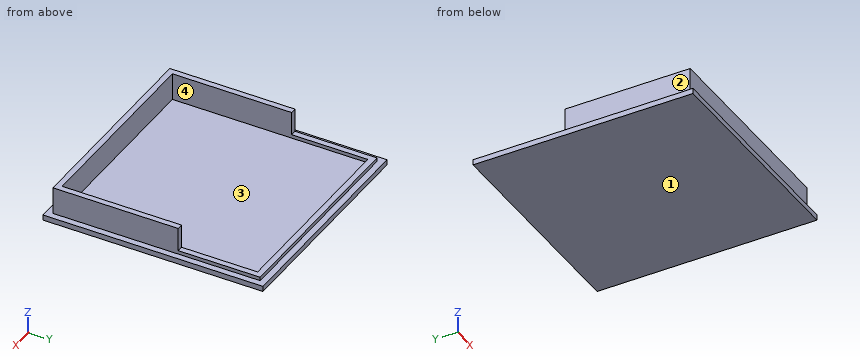
```python
from build123d import *

# Parameters (mm, degrees)
F0_W     = 48.4
F0_H     = 48.4
F3_DEPTH = 1.2
F4_DEPTH = 7.2
F5_DEPTH = 2


with BuildPart() as f3:
    # F0 (on Top) → F3 (new body)
    with BuildSketch(Plane.XY):
        with Locations((0, -0.678107)):
            Rectangle(F0_W, F0_H)
        Polygon((-22.8, 4.06864), (-22.8, 22.121893), (22.8, 22.121893), (22.8, 4.06864), (22.8, -23.478107), (-22.8, -23.478107), align=None, mode=Mode.SUBTRACT)
        Polygon((-21.5, 20.821893), (-21.5, 4.06864), (-21.5, -22.178107), (21.5, -22.178107), (21.5, 4.06864), (21.5, 20.821893), align=None)
        Polygon((22.8, 22.121893), (-22.8, 22.121893), (-22.8, 4.06864), (-21.5, 4.06864), (-21.5, 20.821893), (21.5, 20.821893), (21.5, 4.06864), (22.8, 4.06864), align=None)
        Polygon((-21.5, 4.06864), (-22.8, 4.06864), (-22.8, -23.478107), (22.8, -23.478107), (22.8, 4.06864), (21.5, 4.06864), (21.5, -22.178107), (-21.5, -22.178107), align=None)
    extrude(amount=F3_DEPTH)

    # F1 (on Top) → F4 (join)
    with BuildSketch(Plane.XY):
        Polygon((-21.5, 4.06864), (-22.8, 4.06864), (-22.8, -23.478107), (22.8, -23.478107), (22.8, 4.06864), (21.5, 4.06864), (21.5, -22.178107), (-21.5, -22.178107), align=None)
    extrude(amount=F4_DEPTH)

    # F2 (on Top) → F5 (join)
    with BuildSketch(Plane.XY):
        Polygon((22.8, 22.121893), (-22.8, 22.121893), (-22.8, 4.06864), (-21.5, 4.06864), (-21.5, 20.821893), (21.5, 20.821893), (21.5, 4.06864), (22.8, 4.06864), align=None)
    extrude(amount=F5_DEPTH)


solid = f3.part
```
Can you work these out from the model? Positions are in its coordinate system, mm. Face numbers are marked on the shaded views. Give positions to 0.01 mm unless a question says otherwise; leave off trailing zeros. Order: outer loops, then holes, each group sorted by start corner. A loop starts at its lowest first (then second) coordinate and runs counter-clockwise, first axis right, second up. Notation, with made-up numbers: M 30,-14 L 60,-14 A15 ccw 60,9 Z; hole C 63.5,7.5 d9. An arc over 180 degrees is marked long. One line per item, written item: value.
1) Please list where these lines run through material, in increasing order: line 1 along X through (y, z) = (2.5, 2.75); line 2 along Z through (x, y) = (-18.5, 11); line 3 along Y through (x, z) = (-6.5, 5.25).
Answer sheet:
line 1: x = -22.8 to -21.5, 21.5 to 22.8
line 2: z = 0 to 1.2
line 3: y = -23.48 to -22.18
2) For P1, Ø3, axis at y = -3, z = 3, coming from the -X side; P2, Ø4, axis at x = 8.5, z = 6, coming from the +Y side; P3, Ø3, axis at x = -11.5, y = -11, coming from the +Z side; P4, Ø5, axis at x = -6.5, y = -17.5, coming from the -Z side, each with a flat end and sliding along its axis, tell me the tip position at first contact or that it passes through.
Answer sheet:
P1: stops at x = -22.8
P2: stops at y = -22.18
P3: stops at z = 1.2
P4: stops at z = 0
3) I want a section at C-C, the plane z = 6. List the corners of the cut face in (x, y) for me.
Answer sheet:
outline: M -22.8,-23.48 L 22.8,-23.48 L 22.8,4.07 L 21.5,4.07 L 21.5,-22.18 L -21.5,-22.18 L -21.5,4.07 L -22.8,4.07 Z
4) I want a section at B-B, the plane x = 4. List the corners of the cut face in (y, z) for me, plus the area to 3 significant figures.
Answer sheet:
outline: M -24.88,0 L 23.52,0 L 23.52,1.2 L 22.12,1.2 L 22.12,2 L 20.82,2 L 20.82,1.2 L -22.18,1.2 L -22.18,7.2 L -23.48,7.2 L -23.48,1.2 L -24.88,1.2 Z
area: 66.9 mm^2
5) I want a section at A-A, the plane y = -15.5. List the corners of the cut face in (x, z) for me.
Answer sheet:
outline: M -24.2,0 L 24.2,0 L 24.2,1.2 L 22.8,1.2 L 22.8,7.2 L 21.5,7.2 L 21.5,1.2 L -21.5,1.2 L -21.5,7.2 L -22.8,7.2 L -22.8,1.2 L -24.2,1.2 Z
6) We'd pull the mould along X, two halves only. Please class the marked faces 1, 2, 3 and 4: released by +X, released by -X, zero draft, split by the parting line, or undercut.
Answer sheet:
face 1: zero draft
face 2: released by -X
face 3: undercut
face 4: undercut
